Check sheet for the drawn part. Datum: minimum x, y, z corner. Units: mm. A direction names the side the tool comes from. Round coordinates to 2 decimals unless told otherwise and drop trailing zeros. Loops run counter-clockwise (first coordinate to the right, second up) from the corner with the lowest first, then second, coordinate; pieces in that order, holes last.
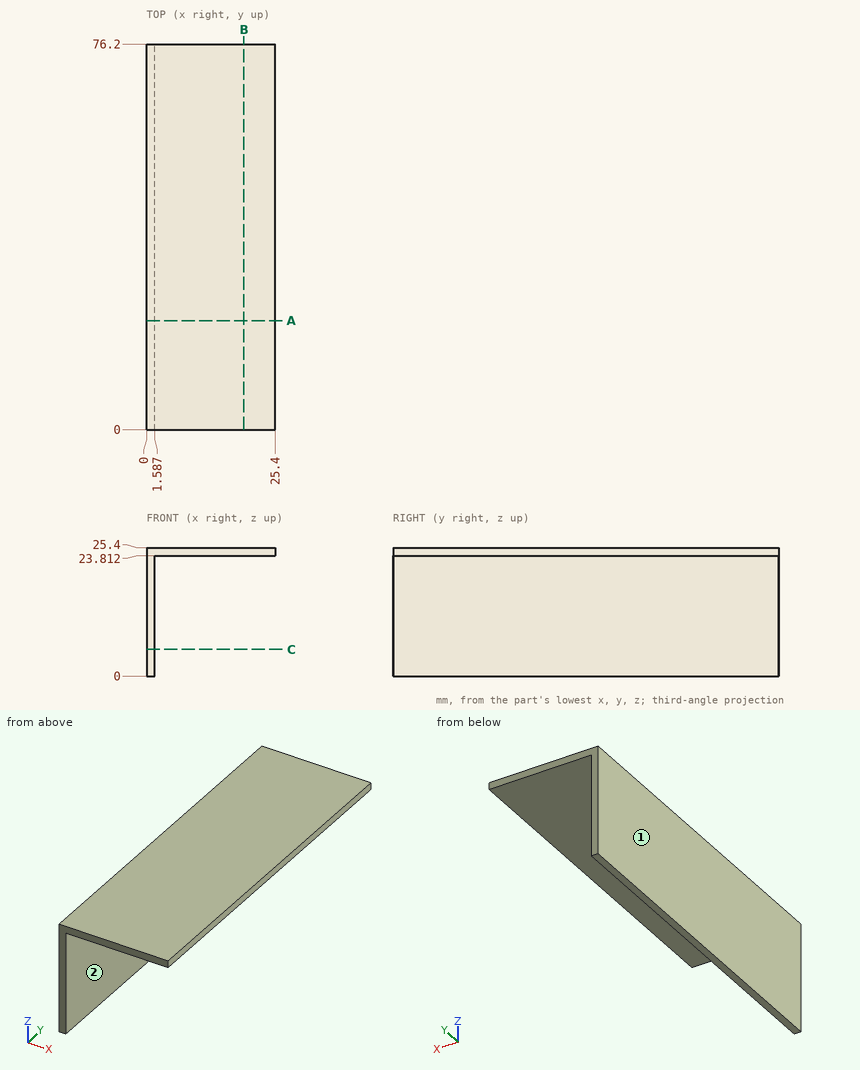
1) Sectioned sample at C-C, the plane z = 5.25. Record the cut outline in (x, y), then the cut area to 3 significant figures.
Report:
outline: (0, 0) - (1.59, 0) - (1.59, 76.2) - (0, 76.2) - close
area: 121 mm2
2) Gauge pin test, flat ends, axial feed: pin 1 (8 mm diameter, centred on y = 19.5, z = 19, fed in from +X); pin 2 (12 mm diameter, centred on x = 11.5, y = 47.5, fed in from -Z); pin 3 (3 mm diameter, centred on x = 11.5, z = 21, fed in from +Y). Record the tip position at first contact, or that the pin passes through.
Report:
pin 1: stops at x = 1.59
pin 2: stops at z = 23.81
pin 3: passes through
3) Sectioned sample at B-B, the plane x = 19.25. Record the cut outline in (y, z), then the cut area to 3 significant figures.
Report:
outline: (0, 23.81) - (76.2, 23.81) - (76.2, 25.4) - (0, 25.4) - close
area: 121 mm2
4) Access from +Z, -Z, +X, -X, +Y, -Y to the whole of each face (thin tool, end or side, straight path). Record for the marked faces 1 and 2.
Report:
face 1: +Z, -Z, -X, +Y, -Y
face 2: -Z, +X, +Y, -Y
5) Sectioned sample at A-A, the plane y = 21.5. Record the cut outline in (x, z).
Report:
outline: (0, 0) - (1.59, 0) - (1.59, 23.81) - (25.4, 23.81) - (25.4, 25.4) - (0, 25.4) - close
6) Scan lines: line 1 along X through (y, z) = (19, 11); line 2 along Z through (x, y) = (6.5, 61.5). Record each from-to range of solid material in increasing order.
Report:
line 1: x = 0 to 1.59
line 2: z = 23.81 to 25.4
